The listing builds one solid part. Answer for the finished solid, in the listing's coordinates (mm). Face numbers are marked on the shaded views. Round coordinates to 2 decimals unless told otherwise and drop trailing zeros. Write each loop counter-clockwise with the first axis right and the second up, starting at its lowest first coordinate (ties: lowest second). Pieces come first, ordered by that corner, then holes.
(1) Find the intervals of material crossed by probe 1 along Y at (x, z) = (-7, -7.25); probe 2 along X at (y, z) = (1.85, -6.25); probe 3 along X at (y, z) = (0.85, 7.5), in increasing order.
(2) Each of these flat-tipped pins is pushed along its axis until it touches: pin 1 Ø1 at (y, z) = (1, -2) entering from -X; pin 2 Ø5.5 at (x, z) = (3.5, 5.5) entering from +Y; pin 3 Ø1.5 at (y, z) = (0.5, 3) entering from -X. Where does it stop, or does it pass through?
(3) A cutting plane is placed at C-C, the plane y = 0.4. Give the vertices of the cut face in (x, z).
(4) A cutting plane is placed at A-A, the plane x = 0. Give the vertices of the cut face in (y, z), and give its area (3 significant figures).
(5) The mould has two halves that part along Z. Classify the marked faces 1 and 2: +Z half, -Z half, draft (parallel to the pull), parting line (faces both ways), or undercut.
(6) A cutting plane is placed at D-D, the plane z = 0. Give the vertices of the cut face in (x, y), and give its area (3 significant figures).
(7) A cutting plane is placed at B-B, the plane z = -7.5. Give the vertices of the cut face in (x, y).
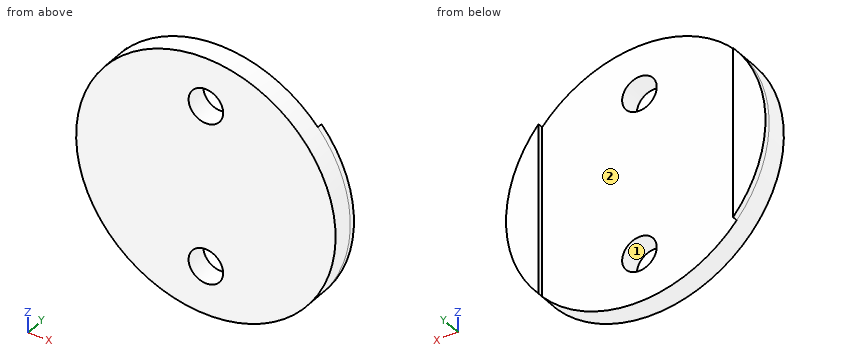
from build123d import *

# Parameters (mm, degrees)
SKETCH_1_R      = 12
SKETCH_1_R_2    = 1.6
EXTRUDE_1_DEPTH = 2
EXTRUDE_2_DEPTH = 0.5


with BuildPart() as part:
    # 草图1 → 凸台-拉伸1 (new body)
    with BuildSketch(Plane(origin=(0, 0, 0), x_dir=(1, 0, 0), z_dir=(0, 1, 0))):
        with Locations(Location((0, 0, 0), (0, 0, 270))):
            Circle(SKETCH_1_R)
        with Locations(Location((0, 7.5, 0), (0, 0, 270))):
            Circle(SKETCH_1_R_2, mode=Mode.SUBTRACT)
        with Locations(Location((0, -7.5, 0), (0, 0, 90))):
            Circle(SKETCH_1_R_2, mode=Mode.SUBTRACT)
    extrude(amount=EXTRUDE_1_DEPTH)

    # 草图2 → 凸台-拉伸2 (add)
    with BuildSketch(Plane(origin=(0, 2, 0), x_dir=(1, 0, 0), z_dir=(0, 1, 0))):
        with BuildLine():
            Line((-9, 7.937253933), (-9, -7.937253933))
            ThreePointArc((-9, -7.937253933), (-12, 0), (-9, 7.937253933))
        make_face()
    extrude_2 = extrude(amount=EXTRUDE_2_DEPTH)

    # 镜向2: 凸台-拉伸2 across plane
    add(extrude_2.mirror(Plane(origin=(0, 0, 0), x_dir=(0, 0, 1), z_dir=(1, 0, 0))))


solid = part.part
Solutions:
1. probe 1: y = 0 to 2
1. probe 2: x = -10.24 to -1, 1 to 10.24
1. probe 3: x = -9.37 to -1.6, 1.6 to 9.37
2. pin 1: stops at x = -11.91
2. pin 2: stops at y = 2
2. pin 3: stops at x = -11.79
3. outline: circle Ø24 at (0, 0); hole circle Ø3.2 at (0, -7.5); hole circle Ø3.2 at (0, 7.5)
4. outline: (0, -12) - (2, -12) - (2, -9.1) - (0, -9.1) - close; (0, -5.9) - (2, -5.9) - (2, 5.9) - (0, 5.9) - close; (0, 9.1) - (2, 9.1) - (2, 12) - (0, 12) - close
4. area: 35.2 mm2
5. face 1: undercut
5. face 2: draft
6. outline: (-12, 0) - (12, 0) - (12, 2.5) - (9, 2.5) - (9, 2) - (-9, 2) - (-9, 2.5) - (-12, 2.5) - close
6. area: 51.0 mm2
7. outline: (-9.37, 0) - (-1.6, 0) - (-1.6, 2) - (-9, 2) - (-9, 2.5) - (-9.37, 2.5) - close; (1.6, 0) - (9.37, 0) - (9.37, 2.5) - (9, 2.5) - (9, 2) - (1.6, 2) - close
